from build123d import *

# Parameters (mm, degrees)
SKETCH1_R            = 7
SKETCH1_R_2          = 4.75
SKETCH1_R_3          = 4
BOSS_EXTRUDE1_DEPTH  = 8
SKETCH1_3_R          = 4.75
SKETCH1_3_R_2        = 4
BOSS_EXTRUDE2_DEPTH  = 80
SKETCH3_R            = 5.75
SKETCH3_R_2          = 3.05
BOSS_EXTRUDE3_DEPTH  = 105
SKETCH8_W            = 50
SKETCH8_H            = 13
BOSS_EXTRUDE8_DEPTH  = 4
SKETCH9_W            = 50
SKETCH9_H            = 6.245985434
BOSS_EXTRUDE9_DEPTH  = 9
BOSS_EXTRUDE10_DEPTH = 50
SKETCH11_W           = 50
SKETCH11_H           = 12.98265639
BOSS_EXTRUDE11_DEPTH = 10
CUT_EXTRUDE1_DEPTH   = 100


with BuildPart() as part:
    # Sketch1 → Boss-Extrude1 (new body)
    # profile 1 of 2: a face of its own
    with BuildSketch(Plane(origin=(0, 0, 0), x_dir=(1, 0, 0), z_dir=(0, 1, 0))):
        with Locations(Location((0, 0, 0), (0, 0, 270))):
            Circle(SKETCH1_R)
        Circle(SKETCH1_R_2, mode=Mode.SUBTRACT)
    # profile 2 of 2: a face of its own
    with BuildSketch(Plane(origin=(0, 0, 0), x_dir=(1, 0, 0), z_dir=(0, 1, 0))):
        Circle(SKETCH1_R_2)
        with Locations(Location((0, 0, 0), (0, 0, 270))):
            Circle(SKETCH1_R_3, mode=Mode.SUBTRACT)
    extrude(amount=BOSS_EXTRUDE1_DEPTH)

    # Sketch1_3 → Boss-Extrude2 (add)
    with BuildSketch(Plane(origin=(0, 0, 0), x_dir=(1, 0, 0), z_dir=(0, 1, 0))):
        with Locations(Location((0, 0, 0), (0, 0, 270))):
            Circle(SKETCH1_3_R)
        with Locations(Location((0, 0, 0), (0, 0, 270))):
            Circle(SKETCH1_3_R_2, mode=Mode.SUBTRACT)
    extrude(amount=BOSS_EXTRUDE2_DEPTH)

    # Sketch3 → Boss-Extrude3 (add)
    with BuildSketch(Plane.XZ):
        with Locations(Location((0, 0, 0), (0, 0, 270))):
            Circle(SKETCH3_R)
        with Locations(Location((0, 0, 0), (0, 0, 270))):
            Circle(SKETCH3_R_2, mode=Mode.SUBTRACT)
    extrude(amount=-BOSS_EXTRUDE3_DEPTH)

    # Sketch8 → Boss-Extrude8 (add)
    with BuildSketch(Plane(origin=(0, 105, 0), x_dir=(1, 0, 0), z_dir=(0, 1, 0))):
        Rectangle(SKETCH8_W, SKETCH8_H)
    extrude(amount=BOSS_EXTRUDE8_DEPTH)

    # Sketch9 → Boss-Extrude9 (add)
    with BuildSketch(Plane(origin=(0, 109, 0), x_dir=(1, 0, 0), z_dir=(0, 1, 0))):
        with Locations((0, -3.377007283)):
            Rectangle(SKETCH9_W, SKETCH9_H)
    extrude(amount=BOSS_EXTRUDE9_DEPTH)

    # Sketch10 → Boss-Extrude10 (add)
    with BuildSketch(Plane.ZY.offset(25)):
        with BuildLine():
            Line((0.254014566, 118), (0.254014566, 109))
            Line((0.254014566, 109), (-6.5, 109))
            ThreePointArc((-6.5, 109), (-4.986953748, 114.898802217), (0.254014566, 118))
        make_face()
    extrude(amount=-BOSS_EXTRUDE10_DEPTH)

    # Sketch11 → Boss-Extrude11 (add)
    with BuildSketch(Plane(origin=(0, 118, 0), x_dir=(1, 0, 0), z_dir=(0, 1, 0))):
        Rectangle(SKETCH11_W, SKETCH11_H)
    extrude(amount=-BOSS_EXTRUDE11_DEPTH)

    # Sketch12 → Cut-Extrude1 (cut)
    with BuildSketch(Plane(origin=(0, 0, -6.491328195), x_dir=(-1, 0, 0), z_dir=(0, 0, -1))):
        with BuildLine():
            Line((-25, 118), (25, 118))
            ThreePointArc((25, 118), (0, 116.124221553), (-25, 118))
        make_face()
    extrude(amount=-CUT_EXTRUDE1_DEPTH, mode=Mode.SUBTRACT)


solid = part.part
Source: CAD feature listing. Evaluate the final solid. Frame: model axes, mm. A direction names the side the tool comes from. Give positions to 0.01 mm unless a question says otherwise; leave off trailing zeros. Write each loop counter-clockwise with the first axis right and the second up, starting at its lowest first coordinate (ties: lowest second). Pieces come first, ordered by that corner, then holes. Notation, with made-up numbers: (69, 41) -> (77, 41) arc R19 ccw to (77, 58) -> close; hole circle Ø5 at (17.25, 40.5). An arc over 180 degrees is marked (long way). Return JSON: item names as keys, results as strings. Group by question number.
1. Section C-C, the plane y = 94. Output: boundary loops of the cut face in (x, z).
2. Access query for faces 1 (the face through (1.5, 0, 3)), 2 (the face through (-1, 8, -6)), 3 (the face through (-6.834, 3.944, -1.517)). Directions: +Z, -Z, +X, -X, +Y, -Y. A direction counts if a zero-diameter tool reaches every point of the face in a straight line with its end or side. Return the directions, or none.
3. Section D-D, the plane x = 17.5. Output: boundary loops of the cut face in (y, z), then the cut area to 3 significant figures.
4. Material intervals for line 1 (X direction, y = 57, z = 0); line 2 (Y direction, x = 0.5, z = 5.25); line 3 (Y direction, x = 0, z = -1.25), sorted ascending. Write a range as from..to.
5. Pin query (flat end, axial travel): pin 1 Ø2 at (x, y) = (-5, 107) entering from -Z; pin 2 Ø5 at (x, z) = (-15, -3.5) entering from -Y; pin 3 Ø1 at (x, z) = (14, -4.5) entering from +Y; pin 4 Ø4 at (x, z) = (-4, -2) entering from -Y. Return the tip coordinate at first contact, or that it passes through.
6. Section A-A, the plane z = 0. Output: boundary loops of the cut face in (x, y).
7. Mould query, pull axis Z, two halves, no side actions, for faces 4 (the face through (-1.856, 51.765, 2.42)), 5 (the face through (25, 112, 0)), 6 (the face through (0, 114, -6.491)). Classes: +Z half, -Z half, draft (parallel to the pull), parting line (faces both ways), or undercut.
8. Section B-B, the plane x = 0. Output: boundary loops of the cut face in (y, z), then the cut area to 3 significant figures.
Determined:
{
 "1": {"outline": "circle Ø11.5 at (0, 0); hole circle Ø6.1 at (0, 0)"},
 "2": {"face 1": "+Z, -Z, +X, -X, -Y", "face 2": "none", "face 3": "-Y"},
 "3": {"outline": "(105, -6.5) -> (109, -6.5) arc R7.96 ccw to (111.31, -6.49) -> (117.04, -6.49) -> (117.04, 6.5) -> (105, 6.5) -> close", "area": "157 mm2"},
 "4": {"line 1": "x = -5.75..-3.05, 3.05..5.75", "line 2": "y = 0..116.12", "line 3": "y = 105..116.12"},
 "5": {"pin 1": "stops at z = -6.5", "pin 2": "stops at y = 105", "pin 3": "stops at y = 116.75", "pin 4": "stops at y = 0"},
 "6": {"outline": "(-25, 105) -> (-5.75, 105) -> (-5.75, 8) -> (-7, 8) -> (-7, 0) -> (-3.05, 0) -> (-3.05, 105) -> (3.05, 105) -> (3.05, 0) -> (7, 0) -> (7, 8) -> (5.75, 8) -> (5.75, 105) -> (25, 105) -> (25, 118) arc R167.54 cw to (-25, 118) -> close"},
 "7": {"face 4": "undercut", "face 5": "draft", "face 6": "-Z half"},
 "8": {"outline": "(0, -7) -> (8, -7) -> (8, -5.75) -> (105, -5.75) -> (105, -6.5) -> (109, -6.5) arc R7.96 ccw to (111.31, -6.49) -> (116.12, -6.49) -> (116.12, 6.5) -> (105, 6.5) -> (105, 5.75) -> (8, 5.75) -> (8, 7) -> (0, 7) -> (0, 3.05) -> (105, 3.05) -> (105, -3.05) -> (0, -3.05) -> close", "area": "732 mm2"}
}
